Build history of the part. All positions in model axes, mm. Face numbers are marked on the shaded views. A direction names the side the tool comes from. Give positions to 0.01 mm unless a question says otherwise; leave off trailing zeros. Order: outer loops, then holes, each group sorted by start corner. A loop starts at its lowest first (then second) coordinate and runs counter-clockwise, first axis right, second up. Notation, with made-up numbers: (49, -16) - (106, -16) arc R12 ccw to (106, 1) - close; hole circle Ø7 at (49.5, 13). An arc over 180 degrees is marked (long way). Use a Markdown table: item, result.
from build123d import *

# Parameters (mm, degrees)
SZKIC1_W                    = 58.4
SZKIC1_H                    = 31.45
DODANIE_WYCI_GNI_CIE1_DEPTH = 4
SZKIC2_W                    = 8.2
SZKIC2_H                    = 5
SZKIC2_W_2                  = 8.7
DODANIE_WYCI_GNI_CIE2_DEPTH = 20.5
WYTNIJ_WYCI_GNI_CIE1_REACH  = 42.563
SZKIC3_R                    = 1.75
SZKIC5_W                    = 58.4
SZKIC5_H                    = 4.2
WYTNIJ_WYCI_GNI_CIE2_DEPTH  = 1.35
SFAZOWANIE1_SIZE            = 2


with BuildPart() as part:
    # Szkic1 → Dodanie-wyciągnięcie1 (new body)
    with BuildSketch(Plane.XY):
        Rectangle(SZKIC1_W, SZKIC1_H)
    extrude(amount=DODANIE_WYCI_GNI_CIE1_DEPTH)

    # Szkic2 → Dodanie-wyciągnięcie2 (add)
    with BuildSketch(Plane(origin=(0, 0, 0), x_dir=(-1, 0, 0), z_dir=(0, 0, -1))):
        with Locations((-25.1, 1.075)):
            Rectangle(SZKIC2_W, SZKIC2_H)
        with Locations((24.85, 1.075)):
            Rectangle(SZKIC2_W_2, SZKIC2_H)
    extrude(amount=DODANIE_WYCI_GNI_CIE2_DEPTH)

    # Szkic3 → Wytnij-wyciągnięcie1 (cut, up to next)
    with BuildSketch(Plane(origin=(0, 3.575, 0), x_dir=(1, 0, 0), z_dir=(0, 1, 0)), mode=Mode.PRIVATE) as wytnij_wyci_gni_cie1_sk1:
        with Locations(Location((25, 4.8, 0), (0, 0, 180))):
            Circle(SZKIC3_R)
    wytnij_wyci_gni_cie1_tool1 = extrude(wytnij_wyci_gni_cie1_sk1.sketch, amount=-WYTNIJ_WYCI_GNI_CIE1_REACH, mode=Mode.PRIVATE) & part.part
    # Szkic3 → Wytnij-wyciągnięcie1 (cut, up to next)
    with BuildSketch(Plane(origin=(0, 3.575, 0), x_dir=(1, 0, 0), z_dir=(0, 1, 0)), mode=Mode.PRIVATE) as wytnij_wyci_gni_cie1_sk2:
        with Locations(Location((-24, 4.8, 0), (0, 0, 180))):
            Circle(SZKIC3_R)
    wytnij_wyci_gni_cie1_tool2 = extrude(wytnij_wyci_gni_cie1_sk2.sketch, amount=-WYTNIJ_WYCI_GNI_CIE1_REACH, mode=Mode.PRIVATE) & part.part
    # Szkic3 → Wytnij-wyciągnięcie1 (cut, up to next)
    with BuildSketch(Plane(origin=(0, 3.575, 0), x_dir=(1, 0, 0), z_dir=(0, 1, 0)), mode=Mode.PRIVATE) as wytnij_wyci_gni_cie1_sk3:
        with Locations(Location((25, 15.7, 0), (0, 0, 270))):
            Circle(SZKIC3_R)
    wytnij_wyci_gni_cie1_tool3 = extrude(wytnij_wyci_gni_cie1_sk3.sketch, amount=-WYTNIJ_WYCI_GNI_CIE1_REACH, mode=Mode.PRIVATE) & part.part
    # Szkic3 → Wytnij-wyciągnięcie1 (cut, up to next)
    with BuildSketch(Plane(origin=(0, 3.575, 0), x_dir=(1, 0, 0), z_dir=(0, 1, 0)), mode=Mode.PRIVATE) as wytnij_wyci_gni_cie1_sk4:
        with Locations(Location((-24, 15.7, 0), (0, 0, 180))):
            Circle(SZKIC3_R)
    wytnij_wyci_gni_cie1_tool4 = extrude(wytnij_wyci_gni_cie1_sk4.sketch, amount=-WYTNIJ_WYCI_GNI_CIE1_REACH, mode=Mode.PRIVATE) & part.part
    add(wytnij_wyci_gni_cie1_tool1.solids().sort_by_distance((25, 3.575, -4.8))[0], mode=Mode.SUBTRACT)
    add(wytnij_wyci_gni_cie1_tool2.solids().sort_by_distance((-24, 3.575, -4.8))[0], mode=Mode.SUBTRACT)
    add(wytnij_wyci_gni_cie1_tool3.solids().sort_by_distance((25, 3.575, -15.7))[0], mode=Mode.SUBTRACT)
    add(wytnij_wyci_gni_cie1_tool4.solids().sort_by_distance((-24, 3.575, -15.7))[0], mode=Mode.SUBTRACT)

    # Szkic5 → Wytnij-wyciągnięcie2 (cut)
    with BuildSketch(Plane(origin=(0, 0, 0), x_dir=(-1, 0, 0), z_dir=(0, 0, -1))):
        with Locations((0, -7.625)):
            Rectangle(SZKIC5_W, SZKIC5_H)
    extrude(amount=-WYTNIJ_WYCI_GNI_CIE2_DEPTH, mode=Mode.SUBTRACT)

    # Sfazowanie1
    sfazowanie1_edges = [part.edges().sort_by_distance(p)[0] for p in [
        (-29.2, 0, 4),
        (29.2, 0, 4),
    ]]
    chamfer(sfazowanie1_edges, length=SFAZOWANIE1_SIZE)


solid = part.part
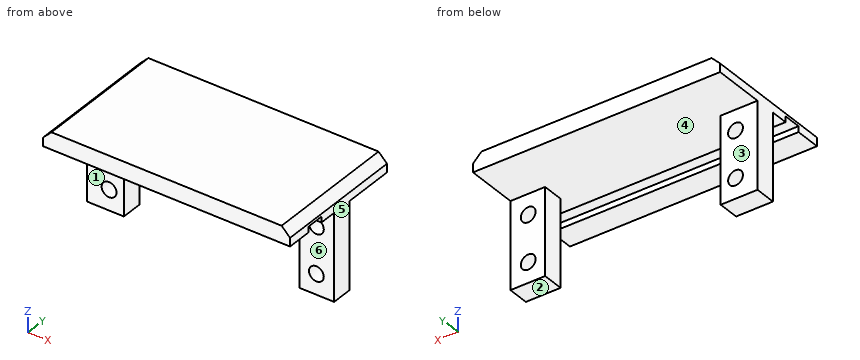
1) Slice it at A-A (z = -4.8). Write the cut outline in (x, y) (3 decimals).
Computed:
| item | result |
|---|---|
| outline | (-29.2, -1.425) - (-25.75, -1.425) - (-25.75, 3.575) - (-29.2, 3.575) - close; (-22.25, -1.425) - (-20.5, -1.425) - (-20.5, 3.575) - (-22.25, 3.575) - close; (21, -1.425) - (23.25, -1.425) - (23.25, 3.575) - (21, 3.575) - close; (26.75, -1.425) - (29.2, -1.425) - (29.2, 3.575) - (26.75, 3.575) - close |
2) Slice it at B-B (y = 0). Write the cut outline in (x, z), and give its area (3 significant figures).
Computed:
| item | result |
|---|---|
| outline | (-29.2, -20.5) - (-20.5, -20.5) - (-20.5, 0) - (21, 0) - (21, -20.5) - (29.2, -20.5) - (29.2, 2) - (27.2, 4) - (-27.2, 4) - (-29.2, 2) - close; hole circle Ø3.5 at (-24, -15.7); hole circle Ø3.5 at (-24, -4.8); hole circle Ø3.5 at (25, -15.7); hole circle Ø3.5 at (25, -4.8) |
| area | 538 mm² |
3) Pin check, flat tips, straight feed: P1, Ø3, axis at x = -24, z = -15.7, coming from the +Y side; P2, Ø7, axis at x = -26, z = -7.5, coming from the +Y side (3 decimals); P3, Ø6.5, axis at x = -11, y = 6.5, coming from the -Z side; P4, Ø12, axis at y = -2, z = -2, coming from the -X side. Stop position of each tip, or through.
Computed:
| item | result |
|---|---|
| P1 | passes through |
| P2 | stops at y = 3.575 |
| P3 | stops at z = 0 |
| P4 | stops at x = -29.2 |
4) Two-plate mould, pull along X, no slides. Class the marked faces 4, 5 and 6: +X half, -X half, draft (parallel to the pull), parting line (faces both ways), or undercut.
Computed:
| item | result |
|---|---|
| face 4 | undercut |
| face 5 | +X half |
| face 6 | draft |
5) Slice it at D-D (z = -12.25). Write the cut outline in (x, y) (3 decimals).
Computed:
| item | result |
|---|---|
| outline | (-29.2, -1.425) - (-20.5, -1.425) - (-20.5, 3.575) - (-29.2, 3.575) - close; (21, -1.425) - (29.2, -1.425) - (29.2, 3.575) - (21, 3.575) - close |
6) Wall check: line 1 (Y direction, x = -5, z = 1.25) (3 decimals); line 2 (Y direction, x = 26, z = -11) (3 decimals); line 3 (Z direction, x = 25, y = -3). Give the ranges that are in metal, low to high. Write a range as from..to.
Computed:
| item | result |
|---|---|
| line 1 | y = -15.725..-9.725, -5.525..15.725 |
| line 2 | y = -1.425..3.575 |
| line 3 | z = 0..4 |
7) Tool access for the marked faces 1, 2 and 3: list every direction of +Z, -Z, +X, -X, +Y, -Y with a clear straight run to the whole face (end or side of a thin tool).
Computed:
| item | result |
|---|---|
| face 1 | -Z, +X, -X, -Y |
| face 2 | -Z, +X, -X, +Y, -Y |
| face 3 | -Z, +X, -X, +Y |
8) Slice it at C-C (x = 25). Write the cut outline in (y, z) (3 decimals).
Computed:
| item | result |
|---|---|
| outline | (-15.725, 0) - (-9.725, 0) - (-9.725, 1.35) - (-5.525, 1.35) - (-5.525, 0) - (-1.425, 0) - (-1.425, -3.05) - (3.575, -3.05) - (3.575, 0) - (15.725, 0) - (15.725, 4) - (-15.725, 4) - close; (-1.425, -20.5) - (3.575, -20.5) - (3.575, -17.45) - (-1.425, -17.45) - close; (-1.425, -13.95) - (3.575, -13.95) - (3.575, -6.55) - (-1.425, -6.55) - close |
